Can you work these out from the model? Positions are in its coordinate system, mm. Round coordinates to 2 decimals unless told otherwise and drop trailing zeros. Write each loop counter-clockwise with the first axis right and the second up, starting at its lowest first coordinate (ties: lowest second). Pieces come first, ordered by that corner, then holes. Notation, with made-up numbers: M 68,15.5 L 100,15.5 A11 cw 100,30.5 Z; hole C 21.5,82.5 d8. An arc over 180 degrees is marked long. Use one line per item in the form item = value. Start each with the question number.
```python
from build123d import *

# Parameters (mm, degrees)
F2_R     = 2.5
F7_DEPTH = 150.001
F8_R     = 25
F9_DEPTH = 75.001


with BuildPart() as f6:
    # F5 (on Right) → F6 (revolve)
    with BuildSketch(Plane.YZ):
        with BuildLine():
            Line((-75, 17.5), (-75, 0))
            Line((-75, 0), (0, 0))
            Line((0, 0), (0, 10))
            ThreePointArc((0, 10), (-37.687034, 11.879664), (-75, 17.5))
        make_face()
        with BuildLine():
            Line((0, 10), (0, 0))
            Line((0, 0), (75, 0))
            Line((75, 0), (75, 17.5))
            ThreePointArc((75, 17.5), (37.687034, 11.879664), (0, 10))
        make_face()
    revolve(axis=Axis((0, 0, 0), (0, 1, 0)))

    # F2 (on offset) → F7 (cut, through all)
    with BuildSketch(Plane.XZ.offset(75)):
        Circle(F2_R)
    extrude(amount=-F7_DEPTH, mode=Mode.SUBTRACT)

    # F8 (on Front) → F9 (cut, through all)
    with BuildSketch(Plane.XZ):
        Circle(F8_R)
    extrude(amount=-F9_DEPTH, mode=Mode.SUBTRACT)


solid = f6.part
```
1. If we section it at A-A (x = 0): List the corners of the cut face in (y, z) for me.
2. Please list where these lines run through material, in increasing order: line 1 along Z through (x, y) = (0, -40); line 2 along Z through (x, y) = (4.5, -69.5); line 3 along Z through (x, y) = (0, -15).
3. If we section it at B-B (z = 0): List the corners of the cut face in (x, y) for me, and give its area (3 significant figures).
4. Will these pins go through, and if not, where does the flat tip stop? pin 1 (3 mm diameter, centred on x = 6.5, y = -9, fed in from -Z); pin 2 (12 mm diameter, centred on y = -43, z = 1.5, fed in from -X); pin 3 (5 mm diameter, centred on x = 5, y = -27.5, fed in from -Z); pin 4 (1 mm diameter, centred on y = -24.5, z = -11.5, fed in from -X).
5. If we section it at D-D (y = -60.5): List the corners of the cut face in (x, z) for me, and give its area (3 significant figures).
6. If we mould it in two halves opening along Z, with no side actions, what happens to faces 1 (the face through (-0.54, -38.02, -2.44)), 2 (the face through (-4, -75, 0))? For each: pulls with the +Z half, pulls with the -Z half, needs draft (parallel to the pull), parting line crosses it, or undercut.
7. If we section it at C-C (y = -50): List the corners of the cut face in (x, z) for me.
Model answer:
q1.outline = M -75,-17.5 A378.75 cw 0,-10 L 0,-2.5 L -75,-2.5 Z; M -75,2.5 L 0,2.5 L 0,10 A378.75 cw -75,17.5 Z
q2.line_1 = -12.12 to -2.5, 2.5 to 12.12
q2.line_2 = -15.8 to 15.8
q2.line_3 = -10.3 to -2.5, 2.5 to 10.3
q3.outline = M -17.5,-75 L -2.5,-75 L -2.5,0 L -10,0 A378.75 cw Z; M 2.5,-75 L 17.5,-75 A378.75 cw 10,0 L 2.5,0 Z
q3.area = 1,500 mm2
q4.pin_1 = -8.78
q4.pin_2 = -13.16
q4.pin_3 = -10.74
q4.pin_4 = through
q5.outline = C 0,0 d29.73; hole C 0,0 d5
q5.area = 674 mm2
q6.face_1 = undercut
q6.face_2 = needs draft
q7.outline = C 0,0 d26.63; hole C 0,0 d5
